Geometry: see drawing. Coordinates: mm, zero at the bounding-box minimum. A direction names the side the tool comes from. Give positions to 0.01 mm unless a question says otherwise; leave off trailing zeros. Write each loop counter-clockwise with the first axis right and the second up, starting at its lowest first coordinate (ties: lowest second). Pieces come first, ordered by that corner, then holes.
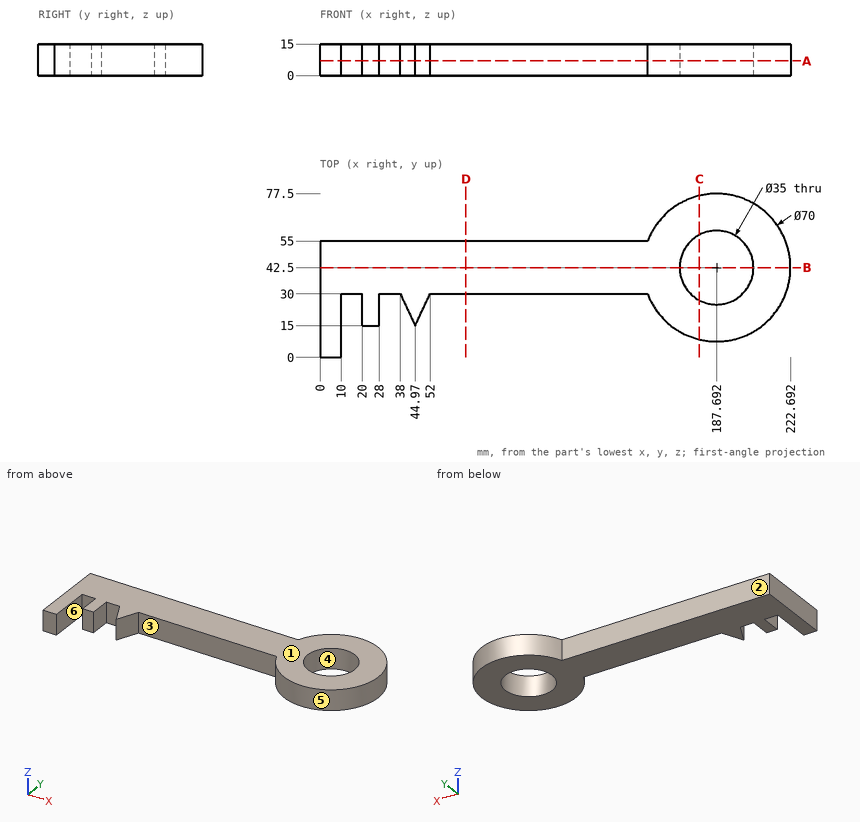
1. Section query D-D (x = 69). Return loops of the section in (y, z), plus the area to 3 significant figures.
2. Section query C-C (x = 179.5). Return loops of the section in (y, z), plus the area to 3 significant figures.
3. Access query for the marked faces 1, 2 and 3. Directions: +Z, -Z, +X, -X, +Y, -Y. A direction counts if a zero-diameter tool reaches every point of the face in a straight line with its end or side. Return the directions, or none.
4. Section query A-A (z = 7). Return loops of the section in (x, y).
5. Pin query (flat end, axial travel): P1, Ø6, axis at y = 57, z = 12, coming from the +X side; P2, Ø4, axis at x = 188.5, z = 6.5, coming from the +Y side; P3, Ø1, axis at y = 63, z = 9.5, coming from the -X side; P4, Ø2, axis at x = 29, y = 14, coming from the +Z side. Return the tip coordinate at first contact, or that it passes through.
6. Section query B-B (y = 42.5). Return loops of the section in (x, z), plus the area to 3 significant figures.
7. Line query: probe 1 along X at (y, z) = (33.5, 3) (1 decimal); probe 2 along X at (y, z) = (12, 12.5) (1 decimal); probe 3 along Y at (x, z) = (128, 8). Output: solid intervals per line, ascending.
8. Pull-direction query (Y, two-part tool) for the marked faces 4, 5 and 6; classes: pulls with the +Y half, pulls with the -Y half, needs draft (parallel to the pull), parting line crosses it, or undercut.
The answers:
1. outline: (30, 0) - (55, 0) - (55, 15) - (30, 15) - close
1. area: 375 mm2
2. outline: (8.47, 0) - (27.04, 0) - (27.04, 15) - (8.47, 15) - close; (57.96, 0) - (76.53, 0) - (76.53, 15) - (57.96, 15) - close
2. area: 557 mm2
3. face 1: +Z, +X, -X, +Y, -Y
3. face 2: +Z, -Z, -X, +Y
3. face 3: +Z, -Z, -Y
4. outline: (0, 0) - (10, 0) - (10, 30) - (20, 30) - (20, 15) - (28, 15) - (28, 30) - (38, 30) - (44.97, 15) - (52, 30) - (155, 30) arc R35 ccw (long way) to (155, 55) - (0, 55) - close; hole circle Ø35 at (187.69, 42.5)
5. P1: stops at x = 220.75
5. P2: stops at y = 77.5
5. P3: stops at x = 158.97
5. P4: passes through
6. outline: (0, 0) - (170.19, 0) - (170.19, 15) - (0, 15) - close; (205.19, 0) - (222.69, 0) - (222.69, 15) - (205.19, 15) - close
6. area: 2,820 mm2
7. probe 1: x = 0 to 172.7, 202.7 to 221.5
7. probe 2: x = 0 to 10, 170.5 to 204.9
7. probe 3: y = 30 to 55
8. face 4: undercut
8. face 5: parting line crosses it
8. face 6: needs draft
